Part model, mm, in its own coordinate system. Round coordinates to 2 decimals unless told otherwise and drop trailing zeros. Loops run counter-clockwise (first coordinate to the right, second up) from the corner with the lowest first, then second, coordinate; pieces in that order, holes last. Notation, with made-up numbers: (63.25, 77.5) - (112.25, 77.5) arc R20 cw to (112.25, 104.5) - close; hole circle Ø1 at (58, -8). An arc over 180 degrees is marked (long way). Write each question's results on one line, items separated by ' | '. Start each with the question number.
(1) Cut at A-A, the plane y = 0. List the corners of the cut face in (x, z), then the cut area to 3 significant figures.
(2) Cut at C-C, the plane x = -23. List the corners of the cut face in (y, z), then the cut area to 3 significant figures.
(3) Flat gauge pins, fed straight in: P1, Ø2, axis at x = -16.5, z = -5, coming from the -Y side; P2, Ø1, axis at y = 3.5, z = 4, coming from the +X side; P3, Ø1, axis at x = -13, z = -5.5, coming from the -Y side (3 decimals); P4, Ø4, axis at y = -0.5, z = 0, coming from the -X side (1 decimal). Where does each tip first touch, or does it go through?
(4) Drill centre lines: L1, parallel to Y at x = -9, z = 0; L2, parallel to X at y = -1.5, z = 5; L3, parallel to Z at x = 17, y = -1. Where is each one in solid material? Low to high.
from build123d import *

# Parameters (mm, degrees)
CUT_EXTRUDE2_REACH = 59.435
SKETCH4_W          = 5
SKETCH4_H          = 5.1
FILLET1_R          = 0.5
SKETCH13_R         = 3.05
CUT_EXTRUDE3_DEPTH = 114.619804612


with BuildPart() as part:
    # Sketch2 → Revolve2 (revolve)
    with BuildSketch(Plane.XY, mode=Mode.PRIVATE) as revolve2_sk:
        Polygon((56.6, 0), (-56.6, 0), (-56.6, 2.55), (-36.2, 2.55), (-36.2, 4.05), (-35, 4.05), (-35, 6.9), (-30, 6.9), (30, 6.9), (35, 6.9), (35, 4.05), (36.2, 4.05), (36.2, 2.55), (56.6, 2.55), align=None)
    revolve(revolve2_sk.sketch.rotate(Axis((62.26, 0, 0), (-1, 0, 0)), 90), axis=Axis((62.26, 0, 0), (-1, 0, 0)))

    # Sketch4 → Cut-Extrude2 (cut, up to next)
    with BuildSketch(Plane(origin=(0, 0, 0), x_dir=(1, 0, 0), z_dir=(0, 1, 0)), mode=Mode.PRIVATE) as cut_extrude2_sk1:
        with Locations((-54.1, 0)):
            Rectangle(SKETCH4_W, SKETCH4_H)
    cut_extrude2_tool1 = extrude(cut_extrude2_sk1.sketch, amount=CUT_EXTRUDE2_REACH, mode=Mode.PRIVATE) & part.part
    add(cut_extrude2_tool1.solids().sort_by_distance((-54.1, 0, 0))[0], mode=Mode.SUBTRACT)

    # Fillet1
    fillet1_edges = [part.edges().sort_by_distance(p)[0] for p in [
        (36.2, 0, 2.55),
        (-36.2, 0, 2.55),
    ]]
    fillet(fillet1_edges, radius=FILLET1_R)

    # Sketch13 → Cut-Extrude3 (cut, through all)
    with BuildSketch(Plane.ZY.offset(56.6)):
        Circle(SKETCH13_R)
    extrude(amount=-CUT_EXTRUDE3_DEPTH, mode=Mode.SUBTRACT)


solid = part.part
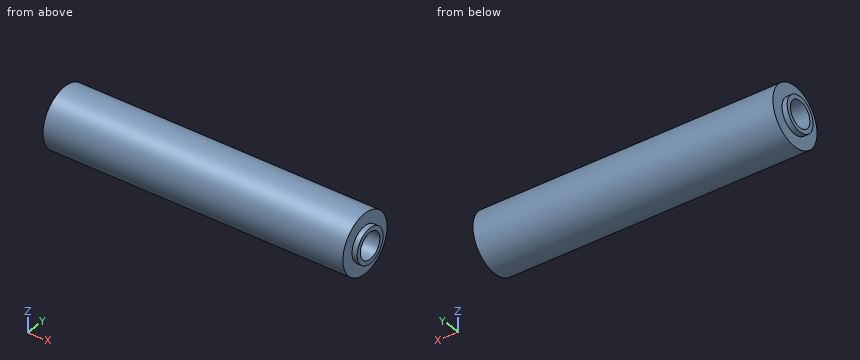
A:
1) outline: (-36.2, -4.05) - (-35, -4.05) - (-35, -6.9) - (35, -6.9) - (35, -4.05) - (36.2, -4.05) - (36.2, -3.05) - (-36.2, -3.05) - close; (-36.2, 3.05) - (36.2, 3.05) - (36.2, 4.05) - (35, 4.05) - (35, 6.9) - (-35, 6.9) - (-35, 4.05) - (-36.2, 4.05) - close | area: 544 mm2
2) outline: circle Ø13.8 at (0, 0); hole circle Ø6.1 at (0, 0) | area: 120 mm2
3) P1: y = -5.62 | P2: x = 35 | P3: y = -4.755 | P4: through
4) L1: -6.9 to -3.05, 3.05 to 6.9 | L2: -35 to 35 | L3: -6.83 to -2.88, 2.88 to 6.83
